For this review, take the finished solid that the model builds, in its own axes (mm). Face numbers are marked on the shaded views. A direction names the side the tool comes from. Coordinates: 2 decimals unless noted, no trailing zeros. Loops run counter-clockwise (first coordinate to the right, second up) from the corner with the lowest first, then second, coordinate; pieces in that order, holes last. Notation, with made-up numbers: M -39.75,37 L 12.25,37 A33 cw 12.25,69 Z; hole C -23.75,21 d8. An arc over 180 degrees is marked long. Write item = value, one per line.
from build123d import *

# Parameters (mm, degrees)
SKETCH1_R           = 12.5
BOSS_EXTRUDE1_DEPTH = 22
SKETCH2_R           = 4.75
BOSS_EXTRUDE2_DEPTH = 7.5
BOSS_EXTRUDE3_DEPTH = 5
BOSS_EXTRUDE4_START = -9.5
SKETCH5_R           = 5
BOSS_EXTRUDE4_DEPTH = 13
SKETCH4_R           = 7.9
SKETCH4_W           = 3
SKETCH4_H           = 38
CUT_EXTRUDE1_DEPTH  = 101.481341552


with BuildPart() as part:
    # Sketch1 → Boss-Extrude1 (new, symmetric)
    with BuildSketch(Plane(origin=(0, 0, 0), x_dir=(0, 0, -1), z_dir=(1, 0, 0))):
        Circle(SKETCH1_R)
    extrude(amount=BOSS_EXTRUDE1_DEPTH, both=True)

    # Sketch2 → Boss-Extrude2 (add, symmetric)
    with BuildSketch(Plane.XY):
        with BuildLine():
            Line((-10, 25), (-10, 0))
            Line((-10, 0), (10, 0))
            Line((10, 0), (10, 25))
            ThreePointArc((10, 25), (0, 35), (-10, 25))
        make_face()
        with Locations((0, 25)):
            Circle(SKETCH2_R, mode=Mode.SUBTRACT)
    extrude(amount=BOSS_EXTRUDE2_DEPTH, both=True)

    # Sketch3 → Boss-Extrude3 (add, symmetric)
    with BuildSketch(Plane.XY):
        with BuildLine():
            Line((-28, -50), (-28, -75))
            Line((-28, -75), (-34, -75))
            Line((-34, -75), (-34, -50))
            ThreePointArc((-34, -50), (-30.01666204, -34.031280577), (-19, -21.80425564))
            Line((-19, -21.80425564), (-19, -8.5))
            Line((-19, -8.5), (19, -8.5))
            Line((19, -8.5), (19, -21.80425564))
            ThreePointArc((19, -21.80425564), (30.01666204, -34.031280577), (34, -50))
            Line((34, -50), (34, -75))
            Line((34, -75), (28, -75))
            Line((28, -75), (28, -50))
            ThreePointArc((28, -50), (0, -22), (-28, -50))
        make_face()
    extrude(amount=BOSS_EXTRUDE3_DEPTH, both=True)

    # Sketch5 → Boss-Extrude4 (add)
    with BuildSketch(Plane(origin=(34, 0, 0), x_dir=(0, 0, -1), z_dir=(1, 0, 0)).offset(BOSS_EXTRUDE4_START)):
        with Locations((0, -75)):
            Circle(SKETCH5_R)
    boss_extrude4 = extrude(amount=BOSS_EXTRUDE4_DEPTH)

    # Mirror1: Boss-Extrude4 across plane
    add(boss_extrude4.mirror(Plane(origin=(0, 0, 0), x_dir=(0, 0, 1), z_dir=(1, 0, 0))))

    # Sketch4 → Cut-Extrude1 (cut, through all)
    with BuildSketch(Plane(origin=(22, 0, 0), x_dir=(0, 0, -1), z_dir=(1, 0, 0))):
        Circle(SKETCH4_R)
        with Locations((0, 19)):
            Rectangle(SKETCH4_W, SKETCH4_H)
    extrude(amount=-CUT_EXTRUDE1_DEPTH, mode=Mode.SUBTRACT)


solid = part.part
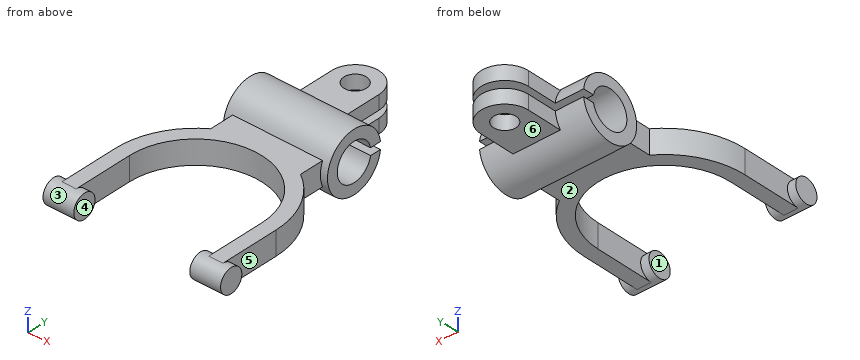
Q1. Machinability: for the marked faces 1, 2 and 3, which of the approach directions +Z, -Z, +X, -X, +Y, -Y give a long, thin tool a straight path to every point of the face, cutting with its end or side? Answer none if there is none.
Solved:
face_1 = +Z, -Z, -Y
face_2 = -Z, +X, -X, -Y
face_3 = none
Q2. For pin 1 Ø5 at (x, z) = (2.5, 0.5) entering from +Y; pin 2 Ø3 at (y, z) = (-60, 2) entering from -X; pin 3 Ø3 at (y, z) = (-26.5, 6) entering from -X; pin 4 Ø5.5 at (x, y) = (0, 25) entering from -Z, all flat-tipped, find the tip position at first contact; note any pin that passes through.
Solved:
pin_1 = 35
pin_2 = -34
pin_3 = -25.59
pin_4 = through
Q3. Add section D-D (y = -60.5). Write out the cut boundary in (x, z), and give its area (3 significant figures).
Solved:
outline = M -34,-5 L -28,-5 L -28,5 L -34,5 Z; M 28,-5 L 34,-5 L 34,5 L 28,5 Z
area = 120 mm²
Q4. Draft analysis for pull direction X (two halves, no side actions). For the marked faces 4, 5 and 6, state which applies: +X half, -X half, draft (parallel to the pull), parting line (faces both ways), or undercut.
Solved:
face_4 = undercut
face_5 = +X half
face_6 = draft
Q5. Add section C-C (z = 0). Write out the cut boundary in (x, y), and give its area (3 significant figures).
Solved:
outline = M -37.5,-80 L -24.5,-80 L -24.5,-70 L -28,-70 L -28,-50 A28 cw 28,-50 L 28,-70 L 24.5,-70 L 24.5,-80 L 37.5,-80 L 37.5,-70 L 34,-70 L 34,-50 A34 ccw 19,-21.8 L 19,-12.5 L 22,-12.5 L 22,-7.9 L -22,-7.9 L -22,-12.5 L -19,-12.5 L -19,-21.8 A34 ccw -34,-50 L -34,-70 L -37.5,-70 Z
area = 1,490 mm²
Q6. For line 1 along Z through (x, y) = (12.5, 0.5); line 2 along X through (y, z) = (25, 5.55); line 3 along X through (y, z) = (-63.5, -4.75), list the stretches that pass through material, from the lowest coordinate up.
Solved:
line_1 = -12.49 to -7.88, 7.88 to 12.49
line_2 = -10 to -4.75, 4.75 to 10
line_3 = -34 to -28, 28 to 34
Q7. Add section B-B (x = 0). Write out the cut boundary in (y, z).
Solved:
outline = M -22,-5 L -11.46,-5 A12.5 ccw 10,-7.5 L 20.25,-7.5 L 20.25,-1.5 L 7.76,-1.5 A7.9 cw long 7.76,1.5 L 20.25,1.5 L 20.25,7.5 L 10,7.5 A12.5 ccw -11.46,5 L -22,5 Z; M 29.75,-7.5 L 35,-7.5 L 35,-1.5 L 29.75,-1.5 Z; M 29.75,1.5 L 35,1.5 L 35,7.5 L 29.75,7.5 Z
Q8. Add section A-A (y = 0). Write out the cut boundary in (x, z), and give its area (3 significant figures).
Solved:
outline = M -22,-12.5 L 22,-12.5 L 22,-7.9 L -22,-7.9 Z; M -22,7.9 L 22,7.9 L 22,12.5 L -22,12.5 Z
area = 405 mm²
